For this review, take the finished solid that the model builds, in its own axes (mm). A direction names the side the tool comes from. Give positions to 0.01 mm unless a question says otherwise; leave off trailing zeros. Order: outer loops, then holes, each group sorted by start corner. A loop starts at its lowest first (then second) coordinate and runs counter-clockwise, first axis right, second up. Notation, with made-up numbers: (10.25, 78.5) -> (25.25, 78.5) arc R19 ccw to (25.25, 91.5) -> close; hole circle Ø11 at (33, 32.25). An arc over 180 degrees is marked (long way). Return JSON: item names as keys, results as strings. Group by question number.
1) For faces 5 (the face through (-17.183, 87.275, -54.563)), 6 (the face through (-58.725, 42, 26)), list the 3-axis set-ups (+Z, -Z, +X, -X, +Y, -Y) from which the entire face can be reached by the end or side of a thin tool; tool diameter is ignored.
2) Add section A-A (y = 87). Give the boundary of the cut face in (x, z), then the cut area to 3 significant figures.
3) Add section B-B (x = -85.5). Give the boundary of the cut face in (y, z), then the cut area to 3 significant figures.
4) Insertion check: P1, Ø1, axis at y = 65.5, z = 9, coming from the +X side; P2, Ø8, axis at y = 44, z = -32, coming from the -X side; P3, Ø1, axis at y = 49.5, z = 33.5, coming from the +X side; P4, Ø5, axis at x = 0, z = 19, coming from the +Y side. Each pin has a flat end and moves straight along its axis. Give the tip position at first contact, or say it passes through.
5) The part is to be moulded in two halves that separate along Y. For faces 1 (the face through (-116.637, -54, 20)), 2 (the face through (-88.086, -2.515, -57.154)), 3 (the face through (-87.28, -55.77, 35.56)), 4 (the face through (-54, 116.637, 20)), say which applies: released by +Y, released by -Y, zero draft, split by the parting line, or undercut.
6) To check wall thickness, follow line 1 along Z through (x, y) = (-14.5, -15); line 2 along Z through (x, y) = (-28, 95.5); line 3 along Y through (x, z) = (-70.5, -36). State the ranges of each line that lie inside material, in increasing order.
from build123d import *

# Parameters (mm, degrees)
SKETCH3_R   = 66.1416
SKETCH3_R_2 = 48.5902


with BuildPart() as part:
    # Sketch1 → Revolve1 (revolve)
    with BuildSketch(Plane.XY, mode=Mode.PRIVATE) as revolve1_sk:
        Polygon((-116.6368, -66.1416), (-58.7248, -66.1416), (-58.7248, -57.0357), (-116.6368, -57.3786), align=None)
    revolve(revolve1_sk.sketch.rotate(Axis((-116.6368, 0, 0), (1, 0, 0)), 270), axis=Axis((-116.6368, 0, 0), (1, 0, 0)))


with BuildPart() as body_2:
    # Sketch2 → Revolve2 (revolve)
    with BuildSketch(Plane.XY, mode=Mode.PRIVATE) as revolve2_sk:
        Polygon((57.3786, 116.6368), (57.0357, 58.7248), (66.1416, 58.7248), (66.1416, 116.6368), align=None)
    revolve(revolve2_sk.sketch.rotate(Axis((0, 0, 0), (0, 1, 0)), 90), axis=Axis((0, 0, 0), (0, 1, 0)))


with BuildPart() as sweep1_tool:
    # Sweep1: sweep along a path in Sketch4
    with BuildLine(Plane.XY) as sweep1_path:
        ThreePointArc((-58.7248, 0), (-17.200096, 17.200096), (0, 58.7248))
    # Sketch3 → Sweep1 (sweep)
    with BuildSketch(Plane(origin=(-58.7248, 0, 0), x_dir=(0, 0, -1), z_dir=(1, 0, 0))):
        Circle(SKETCH3_R)
        Circle(SKETCH3_R_2, mode=Mode.SUBTRACT)
    sweep(path=sweep1_path.line)


with BuildPart() as part_1:
    add(part.part)


with BuildPart() as part_2:
    # Sweep1: joined with sweep1_tool
    add(part_1.part.fuse(sweep1_tool.part, body_2.part, tol=0.00001))


solid = part_2.part
Evaluation:
{
 "1": {"face 5": "+Y", "face 6": "-X"},
 "2": {"outline": "circle Ø132.28 at (0, 0); hole circle Ø114.41 at (0, 0)", "area": "3,460 mm^2"},
 "3": {"outline": "circle Ø132.28 at (0, 0); hole circle Ø114.39 at (0, 0)", "area": "3,470 mm^2"},
 "4": {"P1": "x = 65.59", "P2": "x = -116.64", "P3": "x = 56.96", "P4": "y = -24.2"},
 "5": {"face 1": "zero draft", "face 2": "undercut", "face 3": "split by the parting line", "face 4": "released by +Y"},
 "6": {"line 1": "-60.27 to -40.23, 40.23 to 60.27", "line 2": "-59.92 to -49.94, 49.94 to 59.92", "line 3": "-55.49 to -44.33, 44.33 to 55.49"}
}
